```python
from build123d import *

# Parameters (mm, degrees)
F0_W            = 20
F0_H            = 20
F1_DEPTH        = 413
F2_R            = 2.1
F3_DEPTH        = 413.001
F4_R            = 1
F6_DEPTH        = 413.001
F6_COPIES_COUNT = 4


# Not quite as in the source:
# - a pattern or mirror of a feature is missing from the dataset's text; its kind, count and spacing are read off the source's solid


with BuildPart() as f1:
    # F0 (on Front) → F1 (new body)
    with BuildSketch(Plane.XZ):
        Rectangle(F0_W, F0_H)
    extrude(amount=F1_DEPTH)

    # F2 (on face) → F3 (cut, through all)
    with BuildSketch(Plane.XZ.offset(413)):
        Circle(F2_R)
    extrude(amount=-F3_DEPTH, mode=Mode.SUBTRACT)

    # F4
    f4_edges = [f1.edges().sort_by_distance(p)[0] for p in [
        (-10, -206.5, 10),
        (10, -206.5, 10),
        (10, -206.5, -10),
        (-10, -206.5, -10),
    ]]
    fillet(f4_edges, radius=F4_R)

    # F5 (on face) → F6 (cut, through all)
    with BuildSketch(Plane.XZ.offset(413)):
        Polygon((0, 3.9006601718), (0, 10), (-2.84, 10), (-4.64, 10), (-2.84, 8.2), (-5.4993398282, 8.2), (-5.4993398282, 6.56), (-2.84, 3.9006601718), align=None)
        Polygon((-6.5693398282, 8.2), (-8.2, 8.2), (-7.0953059148, 7.0953059148), (-6.5693398282, 7.6212720014), align=None)
    f6 = extrude(amount=-F6_DEPTH, mode=Mode.SUBTRACT)

    # F6_copies: F6 ×4 about axis
    f6_copies_axis = Axis((0, 0, 0), (0, 1, 0))
    for i in range(1, F6_COPIES_COUNT):
        add(f6.rotate(f6_copies_axis, i * 360 / F6_COPIES_COUNT), mode=Mode.SUBTRACT)

    # F6_copies1: F6 across plane
    add(f6.mirror(Plane(origin=(0, 0, 0), x_dir=(-0.7071067812, 0, -0.7071067812), z_dir=(0.7071067812, 0, -0.7071067812))), mode=Mode.SUBTRACT)

    # F6_copies2: F6 across plane
    add(f6.mirror(Plane(origin=(0, 0, 0), x_dir=(-1, 0, 0), z_dir=(0, 0, -1))), mode=Mode.SUBTRACT)

    # F6_copies3: F6 across plane
    add(f6.mirror(Plane(origin=(0, 0, 0), x_dir=(0, 0, 1), z_dir=(1, 0, 0))), mode=Mode.SUBTRACT)

    # F6_copies4: F6 across plane
    add(f6.mirror(Plane(origin=(0, 0, 0), x_dir=(0.7071067812, 0, -0.7071067812), z_dir=(-0.7071067812, 0, -0.7071067812))), mode=Mode.SUBTRACT)


solid = f1.part
```
Geometry: final body of the model. Coordinates: model frame, mm. Coordinates: 2 decimals unless noted, no trailing zeros. Write each question's results on one line, items separated by ' | '. Start each with the question number.
1) Cut plane A-A, the plane y = -127.5. State how many separate pieces and enclosed holes the cut face has, and give its area (3 significant figures).
2) First-contact query: pin 1 (2 mm diameter, centred on x = 2.5, y = -322, fed in from -Z); pin 2 (6 mm diameter, centred on x = -0.5, y = -185, fed in from +Z); pin 3 (4 mm diameter, centred on y = -109.5, z = 1, fed in from +X). Flat tips, straight axial feed; report the tip coordinate or a pass-through.
3) Material intervals for line 1 along X through (y, z) = (-160.5, 8); line 2 along Z through (x, y) = (0, -314.5); line 3 along Z through (x, y) = (3.5, -272), sorted ascending.
Checks:
1) separate pieces: 1 | enclosed holes: 5 | area: 162 mm^2
2) pin 1: z = -8.86 | pin 2: z = 8.86 | pin 3: x = 8.36
3) line 1: -10 to -8.2, -6.57 to -5.5, 5.5 to 6.57, 8.2 to 10 | line 2: -3.9 to -2.1, 2.1 to 3.9 | line 3: -8.86 to -8.2, -4.56 to 4.56, 8.2 to 8.86
